```python
from build123d import *

# Parameters (mm, degrees)
SKETCH_1_R          = 10.65
SKETCH_1_R_2        = 3.5
EXTRUDE_1_DEPTH     = 2
SKETCH_2_R          = 4.3
SKETCH_2_R_2        = 3
EXTRUDE_2_DEPTH     = 3.8
FILLET_1_R          = 1
CUT_EXTRUDE_1_REACH = 7.8
SKETCH_3_R          = 0.8


with BuildPart() as part:
    # Эскиз1 → Бобышка-Вытянуть1 (new body)
    with BuildSketch(Plane(origin=(0, 0, 0), x_dir=(1, 0, 0), z_dir=(0, 1, 0))):
        Circle(SKETCH_1_R)
        Circle(SKETCH_1_R_2, mode=Mode.SUBTRACT)
    extrude(amount=EXTRUDE_1_DEPTH)

    # Эскиз2 → Бобышка-Вытянуть2 (add)
    with BuildSketch(Plane.XZ):
        Circle(SKETCH_2_R)
        Circle(SKETCH_2_R_2, mode=Mode.SUBTRACT)
    extrude(amount=EXTRUDE_2_DEPTH)

    # Скругление1
    fillet_1_edges = [part.edges().sort_by_distance(p)[0] for p in [
        (-4.3, 0, 0),
    ]]
    fillet(fillet_1_edges, radius=FILLET_1_R)

    # Эскиз3 → Вырез-Вытянуть1 (cut, up to next)
    with BuildSketch(Plane(origin=(0, 2, 0), x_dir=(1, 0, 0), z_dir=(0, 1, 0)), mode=Mode.PRIVATE) as cut_extrude_1_sk1:
        with Locations((-3.5, 7.5)):
            Circle(SKETCH_3_R)
    cut_extrude_1_tool1 = extrude(cut_extrude_1_sk1.sketch, amount=-CUT_EXTRUDE_1_REACH, mode=Mode.PRIVATE) & part.part
    add(cut_extrude_1_tool1.solids().sort_by_distance((-3.5, 2, -7.5))[0], mode=Mode.SUBTRACT)
    # Эскиз3 → Вырез-Вытянуть1 (cut, up to next)
    with BuildSketch(Plane(origin=(0, 2, 0), x_dir=(1, 0, 0), z_dir=(0, 1, 0)), mode=Mode.PRIVATE) as cut_extrude_1_sk2:
        with Locations((0, 7.5)):
            Circle(SKETCH_3_R)
    cut_extrude_1_tool2 = extrude(cut_extrude_1_sk2.sketch, amount=-CUT_EXTRUDE_1_REACH, mode=Mode.PRIVATE) & part.part
    add(cut_extrude_1_tool2.solids().sort_by_distance((0, 2, -7.5))[0], mode=Mode.SUBTRACT)
    # Эскиз3 → Вырез-Вытянуть1 (cut, up to next)
    with BuildSketch(Plane(origin=(0, 2, 0), x_dir=(1, 0, 0), z_dir=(0, 1, 0)), mode=Mode.PRIVATE) as cut_extrude_1_sk3:
        with Locations((3.5, 7.5)):
            Circle(SKETCH_3_R)
    cut_extrude_1_tool3 = extrude(cut_extrude_1_sk3.sketch, amount=-CUT_EXTRUDE_1_REACH, mode=Mode.PRIVATE) & part.part
    add(cut_extrude_1_tool3.solids().sort_by_distance((3.5, 2, -7.5))[0], mode=Mode.SUBTRACT)
    # Эскиз3 → Вырез-Вытянуть1 (cut, up to next)
    with BuildSketch(Plane(origin=(0, 2, 0), x_dir=(1, 0, 0), z_dir=(0, 1, 0)), mode=Mode.PRIVATE) as cut_extrude_1_sk4:
        with Locations((7.5, 3.5)):
            Circle(SKETCH_3_R)
    cut_extrude_1_tool4 = extrude(cut_extrude_1_sk4.sketch, amount=-CUT_EXTRUDE_1_REACH, mode=Mode.PRIVATE) & part.part
    add(cut_extrude_1_tool4.solids().sort_by_distance((7.5, 2, -3.5))[0], mode=Mode.SUBTRACT)
    # Эскиз3 → Вырез-Вытянуть1 (cut, up to next)
    with BuildSketch(Plane(origin=(0, 2, 0), x_dir=(1, 0, 0), z_dir=(0, 1, 0)), mode=Mode.PRIVATE) as cut_extrude_1_sk5:
        with Locations((7.5, 0)):
            Circle(SKETCH_3_R)
    cut_extrude_1_tool5 = extrude(cut_extrude_1_sk5.sketch, amount=-CUT_EXTRUDE_1_REACH, mode=Mode.PRIVATE) & part.part
    add(cut_extrude_1_tool5.solids().sort_by_distance((7.5, 2, 0))[0], mode=Mode.SUBTRACT)
    # Эскиз3 → Вырез-Вытянуть1 (cut, up to next)
    with BuildSketch(Plane(origin=(0, 2, 0), x_dir=(1, 0, 0), z_dir=(0, 1, 0)), mode=Mode.PRIVATE) as cut_extrude_1_sk6:
        with Locations((7.5, -3.5)):
            Circle(SKETCH_3_R)
    cut_extrude_1_tool6 = extrude(cut_extrude_1_sk6.sketch, amount=-CUT_EXTRUDE_1_REACH, mode=Mode.PRIVATE) & part.part
    add(cut_extrude_1_tool6.solids().sort_by_distance((7.5, 2, 3.5))[0], mode=Mode.SUBTRACT)
    # Эскиз3 → Вырез-Вытянуть1 (cut, up to next)
    with BuildSketch(Plane(origin=(0, 2, 0), x_dir=(1, 0, 0), z_dir=(0, 1, 0)), mode=Mode.PRIVATE) as cut_extrude_1_sk7:
        with Locations((3.5, -7.5)):
            Circle(SKETCH_3_R)
    cut_extrude_1_tool7 = extrude(cut_extrude_1_sk7.sketch, amount=-CUT_EXTRUDE_1_REACH, mode=Mode.PRIVATE) & part.part
    add(cut_extrude_1_tool7.solids().sort_by_distance((3.5, 2, 7.5))[0], mode=Mode.SUBTRACT)
    # Эскиз3 → Вырез-Вытянуть1 (cut, up to next)
    with BuildSketch(Plane(origin=(0, 2, 0), x_dir=(1, 0, 0), z_dir=(0, 1, 0)), mode=Mode.PRIVATE) as cut_extrude_1_sk8:
        with Locations((0, -7.5)):
            Circle(SKETCH_3_R)
    cut_extrude_1_tool8 = extrude(cut_extrude_1_sk8.sketch, amount=-CUT_EXTRUDE_1_REACH, mode=Mode.PRIVATE) & part.part
    add(cut_extrude_1_tool8.solids().sort_by_distance((0, 2, 7.5))[0], mode=Mode.SUBTRACT)
    # Эскиз3 → Вырез-Вытянуть1 (cut, up to next)
    with BuildSketch(Plane(origin=(0, 2, 0), x_dir=(1, 0, 0), z_dir=(0, 1, 0)), mode=Mode.PRIVATE) as cut_extrude_1_sk9:
        with Locations((-3.5, -7.5)):
            Circle(SKETCH_3_R)
    cut_extrude_1_tool9 = extrude(cut_extrude_1_sk9.sketch, amount=-CUT_EXTRUDE_1_REACH, mode=Mode.PRIVATE) & part.part
    add(cut_extrude_1_tool9.solids().sort_by_distance((-3.5, 2, 7.5))[0], mode=Mode.SUBTRACT)
    # Эскиз3 → Вырез-Вытянуть1 (cut, up to next)
    with BuildSketch(Plane(origin=(0, 2, 0), x_dir=(1, 0, 0), z_dir=(0, 1, 0)), mode=Mode.PRIVATE) as cut_extrude_1_sk10:
        with Locations((-7.5, -3.5)):
            Circle(SKETCH_3_R)
    cut_extrude_1_tool10 = extrude(cut_extrude_1_sk10.sketch, amount=-CUT_EXTRUDE_1_REACH, mode=Mode.PRIVATE) & part.part
    add(cut_extrude_1_tool10.solids().sort_by_distance((-7.5, 2, 3.5))[0], mode=Mode.SUBTRACT)
    # Эскиз3 → Вырез-Вытянуть1 (cut, up to next)
    with BuildSketch(Plane(origin=(0, 2, 0), x_dir=(1, 0, 0), z_dir=(0, 1, 0)), mode=Mode.PRIVATE) as cut_extrude_1_sk11:
        with Locations((-7.5, 0)):
            Circle(SKETCH_3_R)
    cut_extrude_1_tool11 = extrude(cut_extrude_1_sk11.sketch, amount=-CUT_EXTRUDE_1_REACH, mode=Mode.PRIVATE) & part.part
    add(cut_extrude_1_tool11.solids().sort_by_distance((-7.5, 2, 0))[0], mode=Mode.SUBTRACT)
    # Эскиз3 → Вырез-Вытянуть1 (cut, up to next)
    with BuildSketch(Plane(origin=(0, 2, 0), x_dir=(1, 0, 0), z_dir=(0, 1, 0)), mode=Mode.PRIVATE) as cut_extrude_1_sk12:
        with Locations((-7.5, 3.5)):
            Circle(SKETCH_3_R)
    cut_extrude_1_tool12 = extrude(cut_extrude_1_sk12.sketch, amount=-CUT_EXTRUDE_1_REACH, mode=Mode.PRIVATE) & part.part
    add(cut_extrude_1_tool12.solids().sort_by_distance((-7.5, 2, -3.5))[0], mode=Mode.SUBTRACT)


solid = part.part
```
Here's how the part is built. I have some questions about the finished solid (model axes, mm). A direction names the side the tool comes from. Coordinates: 2 decimals unless noted, no trailing zeros. Order: outer loops, then holes, each group sorted by start corner. A loop starts at its lowest first (then second) coordinate and runs counter-clockwise, first axis right, second up. Notation, with made-up numbers: (66.5, 69.25) - (75.5, 69.25) arc R26 ccw to (75.5, 103.25) - close; hole circle Ø1 at (33, -15). An arc over 180 degrees is marked (long way). One line per question, with ' | ' between items.
(1) Suppose I cut it at A-A on x = 0. List the corners of the cut face in (y, z) for me.
Report:
outline: (-3.8, -4.3) - (-1, -4.3) arc R1 cw to (0, -5.3) - (0, -6.7) - (2, -6.7) - (2, -3.5) - (0, -3.5) - (0, -3) - (-3.8, -3) - close; (-3.8, 3) - (0, 3) - (0, 3.5) - (2, 3.5) - (2, 6.7) - (0, 6.7) - (0, 5.3) arc R1 cw to (-1, 4.3) - (-3.8, 4.3) - close; (0, -10.65) - (2, -10.65) - (2, -8.3) - (0, -8.3) - close; (0, 8.3) - (2, 8.3) - (2, 10.65) - (0, 10.65) - close
(2) Suppose I cut it at B-B on z = 7.5. List the corners of the cut face in (x, y) for me, and give its area (3 significant figures).
Report:
outline: (-7.56, 0) - (-4.3, 0) - (-4.3, 2) - (-7.56, 2) - close; (-2.7, 0) - (-0.8, 0) - (-0.8, 2) - (-2.7, 2) - close; (0.8, 0) - (2.7, 0) - (2.7, 2) - (0.8, 2) - close; (4.3, 0) - (7.56, 0) - (7.56, 2) - (4.3, 2) - close | area: 20.6 mm2
(3) Suppose I cut it at C-C on y = -0.4. List the corners of the cut face in (x, z) for me.
Report:
outline: circle Ø9 at (0, 0); hole circle Ø6 at (0, 0)
(4) Suppose I cut it at D-D on x = 7.5. List the corners of the cut face in (y, z) for me.
Report:
outline: (0, -7.56) - (2, -7.56) - (2, -4.3) - (0, -4.3) - close; (0, -2.7) - (2, -2.7) - (2, -0.8) - (0, -0.8) - close; (0, 0.8) - (2, 0.8) - (2, 2.7) - (0, 2.7) - close; (0, 4.3) - (2, 4.3) - (2, 7.56) - (0, 7.56) - close
(5) If we mould it in two halves opening along Z, with no side actions, what happens to faces 4 (the flat face through (-3, -3.8, -1)), 5 (the cylindrical face through (-8.3, 1, 0)), 6 (the cylindrical face through (10.158, 0.986, -3.199))? For each: pulls with the +Z half, pulls with the -Z half, needs draft (parallel to the pull), parting line crosses it, or undercut.
Report:
face 4: needs draft | face 5: undercut | face 6: parting line crosses it
(6) Will these pins go through, and if not, where does the flat tip stop? pin 1 (7 mm diameter, centred on x = 0, z = 0, fed in from -Y); pin 2 (2 mm diameter, centred on x = -8, z = -8, fed in from -Y); pin 3 (1.3 mm diameter, centred on x = -3.5, z = -7.5, fed in from -Y); pin 4 (2 mm diameter, centred on x = -2, z = -5.5, fed in from -Y).
Report:
pin 1: stops at y = -3.8 | pin 2: stops at y = 0 | pin 3: passes through | pin 4: stops at y = -0.11
(7) If I drill on L1, parallel to Z at x = 0, y = 0.85; L2, parallel to Z at x = 7.5, y = 1.6, over which ranges is the centre line in solid material (lowest first)?
Report:
L1: z = -10.65 to -8.3, -6.7 to -3.5, 3.5 to 6.7, 8.3 to 10.65 | L2: z = -7.56 to -4.3, -2.7 to -0.8, 0.8 to 2.7, 4.3 to 7.56
(8) For faces 1 (the cylindrical face through (3.396, 1.014, -8.293)), 2 (the cylindrical face through (-4.296, -2.38, 0.189)), 3 (the flat face through (3, 0, 1)), which set-ups out of +Z, -Z, +X, -X, +Y, -Y let a thin tool reach every point of the face, with its end or its side?
Report:
face 1: +Y, -Y | face 2: -Y | face 3: +Y
